```python
from build123d import *

# Parameters (mm, degrees)
BOX100_W                  = 187
BOX100_H                  = 3.4
BOX100_DEPTH              = 115
CYLINDER175_R             = 3
CYLINDER175_DEPTH         = 200
CYLINDER175_ROLL_ANGLE    = 90
CYLINDER176_R             = 3
CYLINDER176_DEPTH         = 200
CYLINDER176_ROLL_ANGLE    = 90
CYLINDER178_R             = 1.5
CYLINDER178_DEPTH         = 200
CYLINDER178_ROLL_ANGLE    = 90
CYLINDER177_R             = 1.5
CYLINDER177_DEPTH         = 200
CYLINDER177_ROLL_ANGLE    = 90
PAD090_DEPTH              = 55
BOX094_W                  = 5
BOX094_H                  = 176
BOX094_DEPTH              = 140
PAD091_DEPTH              = 55
BOX095_W                  = 6
BOX095_H                  = 176
BOX095_DEPTH              = 140
BOX093_W                  = 33
BOX093_H                  = 132
BOX093_DEPTH              = 54
BOX093_PLACEMENT_ANGLE    = 3
FILLET087_R               = 10
FILLET087_PLACEMENT_ANGLE = -3
BOX091_W                  = 18
BOX091_H                  = 17
BOX091_DEPTH              = 140
FILLET086_R               = 10
BOX090_W                  = 18
BOX090_H                  = 17
BOX090_DEPTH              = 140
FILLET085_R               = 10
BOX092_W                  = 182
BOX092_H                  = 16
BOX092_DEPTH              = 35
BOX097_W                  = 6
BOX097_H                  = 176
BOX097_DEPTH              = 80
BOX096_W                  = 5
BOX096_H                  = 176
BOX096_DEPTH              = 80
BOX088_W                  = 218
BOX088_H                  = 197
BOX088_DEPTH              = 10
FILLET083_R               = 10
FILLET084_R               = 10
CYLINDER172_R             = 2
CYLINDER172_DEPTH         = 300
CYLINDER172_PITCH_ANGLE   = 90
BOX099_W                  = 60
BOX099_H                  = 10
BOX099_DEPTH              = 10
FILLET089_R               = 4
FILLET090_R               = 10
FILLET091_R               = 10


with BuildPart() as cubo095:
    # Box100 → Box100 (new body)
    with BuildSketch(Plane(origin=(0, -44, 0), x_dir=(1, 0, 0), z_dir=(0, 0, 1))):
        with Locations((93.5, 1.7)):
            Rectangle(BOX100_W, BOX100_H)
    extrude(amount=BOX100_DEPTH)


with BuildPart() as obj1:
    # Cylinder175 → Cylinder175 (new body)
    with BuildSketch(Plane.XY):
        Circle(CYLINDER175_R)
    extrude(amount=CYLINDER175_DEPTH)


with BuildPart() as obj1_1:
    # Cylinder175 roll: moved
    add(obj1.part.rotate(Axis((0, 0, 0), (1, 0, 0)), CYLINDER175_ROLL_ANGLE))


with BuildPart() as obj1_2:
    # Cylinder175 placement: moved
    add(obj1_1.part.moved(Location((20, 165, 110))))


with BuildPart() as obj2:
    # Cylinder176 → Cylinder176 (new body)
    with BuildSketch(Plane.XY):
        Circle(CYLINDER176_R)
    extrude(amount=CYLINDER176_DEPTH)


with BuildPart() as obj2_1:
    # Cylinder176 roll: moved
    add(obj2.part.rotate(Axis((0, 0, 0), (1, 0, 0)), CYLINDER176_ROLL_ANGLE))


with BuildPart() as obj2_2:
    # Cylinder176 placement: moved
    add(obj2_1.part.moved(Location((160, 165, 110))))


with BuildPart() as obj3:
    # Cylinder178 → Cylinder178 (new body)
    with BuildSketch(Plane.XY):
        Circle(CYLINDER178_R)
    extrude(amount=CYLINDER178_DEPTH)


with BuildPart() as obj3_1:
    # Cylinder178 roll: moved
    add(obj3.part.rotate(Axis((0, 0, 0), (1, 0, 0)), CYLINDER178_ROLL_ANGLE))


with BuildPart() as obj3_2:
    # Cylinder178 placement: moved
    add(obj3_1.part.moved(Location((160, 154, 110))))


with BuildPart() as obj4:
    # Cylinder177 → Cylinder177 (new body)
    with BuildSketch(Plane.XY):
        Circle(CYLINDER177_R)
    extrude(amount=CYLINDER177_DEPTH)


with BuildPart() as obj4_1:
    # Cylinder177 roll: moved
    add(obj4.part.rotate(Axis((0, 0, 0), (1, 0, 0)), CYLINDER177_ROLL_ANGLE))


with BuildPart() as obj4_2:
    # Cylinder177 placement: moved
    add(obj4_1.part.moved(Location((20, 154, 110))))


with BuildPart() as pad090:
    # Sketch098 → Pad090 (new body)
    with BuildSketch(Plane(origin=(0, 0, 0), x_dir=(0, -1, 0), z_dir=(-1, 0, 0))):
        Polygon((-174.561249, 149.464645), (-73.728157, 149.464645), (-50.393822, 111), (-27.455967, 92.725647), (51.678024, 92.725647), (59.260941, 172), (-154.48703, 174.345367), align=None)
    extrude(amount=PAD090_DEPTH)


with BuildPart() as cut209:
    # Box094 → Box094 (new body)
    with BuildSketch(Plane(origin=(-15, -35, 0), x_dir=(1, 0, 0), z_dir=(0, 0, 1))):
        with Locations((2.5, 88)):
            Rectangle(BOX094_W, BOX094_H)
    extrude(amount=BOX094_DEPTH)

    # Cut209: cut Pad090
    add(pad090.part, mode=Mode.SUBTRACT)


with BuildPart() as pad091:
    # Sketch099 → Pad091 (new body)
    with BuildSketch(Plane(origin=(0, 0, 0), x_dir=(0, -1, 0), z_dir=(-1, 0, 0))):
        Polygon((-174.561249, 149.464645), (-73.728157, 149.464645), (-50.393822, 111), (-27.455967, 92.725647), (51.678024, 92.725647), (59.260941, 172), (-154.48703, 174.345367), align=None)
    extrude(amount=PAD091_DEPTH)


with BuildPart() as cut210:
    # Box095 → Box095 (new body)
    with BuildSketch(Plane(origin=(-15, -35, 0), x_dir=(1, 0, 0), z_dir=(0, 0, 1))):
        with Locations((3, 88)):
            Rectangle(BOX095_W, BOX095_H)
    extrude(amount=BOX095_DEPTH)

    # Cut210: cut Pad091
    add(pad091.part, mode=Mode.SUBTRACT)


with BuildPart() as cut210_1:
    # Cut210 placement: moved
    add(cut210.part.moved(Location((212, 0, 0))))


with BuildPart() as fillet104:
    # Box093 → Box093 (new body)
    with BuildSketch(Plane.XY):
        with Locations((16.5, 66)):
            Rectangle(BOX093_W, BOX093_H)
    extrude(amount=BOX093_DEPTH)


with BuildPart() as fillet104_1:
    # Box093 placement: moved
    add(fillet104.part.moved(Location((188, -32, 69))).rotate(Axis((188, -32, 69), (0, 0, 1)), BOX093_PLACEMENT_ANGLE))

    # Fillet087
    fillet087_edges = [fillet104_1.edges().sort_by_distance(p)[0] for p in [
        (204.477387, -31.136457, 69),
        (204.477387, -31.136457, 123),
        (197.569041, 100.682642, 69),
        (197.569041, 100.682642, 123),
    ]]
    fillet(fillet087_edges, radius=FILLET087_R)


with BuildPart() as fillet104_2:
    # Fillet087 placement: moved
    add(fillet104_1.part.moved(Location((0, 12, 0))).rotate(Axis((0, 12, 0), (0, 0, 1)), FILLET087_PLACEMENT_ANGLE))


with BuildPart() as fillet103:
    # Box091 → Box091 (new body)
    with BuildSketch(Plane(origin=(185, -48, 0), x_dir=(1, 0, 0), z_dir=(0, 0, 1))):
        with Locations((9, 8.5)):
            Rectangle(BOX091_W, BOX091_H)
    extrude(amount=BOX091_DEPTH)

    # Fillet086
    fillet086_edges = [fillet103.edges().sort_by_distance(p)[0] for p in [
        (203, -48, 70),
    ]]
    fillet(fillet086_edges, radius=FILLET086_R)


with BuildPart() as fillet102:
    # Box090 → Box090 (new body)
    with BuildSketch(Plane(origin=(-15, -48, 0), x_dir=(1, 0, 0), z_dir=(0, 0, 1))):
        with Locations((9, 8.5)):
            Rectangle(BOX090_W, BOX090_H)
    extrude(amount=BOX090_DEPTH)

    # Fillet085
    fillet085_edges = [fillet102.edges().sort_by_distance(p)[0] for p in [
        (-15, -48, 70),
    ]]
    fillet(fillet085_edges, radius=FILLET085_R)


with BuildPart() as cubo087:
    # Box092 → Box092 (new body)
    with BuildSketch(Plane(origin=(3, -48, 105), x_dir=(1, 0, 0), z_dir=(0, 0, 1))):
        with Locations((91, 8)):
            Rectangle(BOX092_W, BOX092_H)
    extrude(amount=BOX092_DEPTH)


with BuildPart() as cubo092:
    # Box097 → Box097 (new body)
    with BuildSketch(Plane(origin=(197, -35, 61), x_dir=(1, 0, 0), z_dir=(0, 0, 1))):
        with Locations((3, 88)):
            Rectangle(BOX097_W, BOX097_H)
    extrude(amount=BOX097_DEPTH)


with BuildPart() as cubo091:
    # Box096 → Box096 (new body)
    with BuildSketch(Plane(origin=(-15, -35, 61), x_dir=(1, 0, 0), z_dir=(0, 0, 1))):
        with Locations((2.5, 88)):
            Rectangle(BOX096_W, BOX096_H)
    extrude(amount=BOX096_DEPTH)


with BuildPart() as cut213:
    # Box088 → Box088 (new body)
    with BuildSketch(Plane(origin=(-15, -48, 140), x_dir=(1, 0, 0), z_dir=(0, 0, 1))):
        with Locations((109, 98.5)):
            Rectangle(BOX088_W, BOX088_H)
    extrude(amount=BOX088_DEPTH)

    # Fillet083
    fillet083_edges = [cut213.edges().sort_by_distance(p)[0] for p in [
        (-15, 149, 145),
        (203, 149, 145),
    ]]
    fillet(fillet083_edges, radius=FILLET083_R)

    # Fillet084
    fillet084_edges = [cut213.edges().sort_by_distance(p)[0] for p in [
        (-15, -48, 145),
        (203, -48, 145),
    ]]
    fillet(fillet084_edges, radius=FILLET084_R)

    # Fusion092: union Cubo092, Cubo091
    add(cubo092.part)
    add(cubo091.part)

    # Fusion093: union Fillet103, Fillet102, Cubo087
    add(fillet103.part)
    add(fillet102.part)
    add(cubo087.part)

    # Cut211: cut Fillet104
    add(fillet104_2.part, mode=Mode.SUBTRACT)

    # Cut212: cut Cut210
    add(cut210_1.part, mode=Mode.SUBTRACT)

    # Cut213: cut Cut209
    add(cut209.part, mode=Mode.SUBTRACT)


with BuildPart() as obj5:
    # Cylinder172 → Cylinder172 (new body)
    with BuildSketch(Plane.XY):
        Circle(CYLINDER172_R)
    extrude(amount=CYLINDER172_DEPTH)


with BuildPart() as obj5_1:
    # Cylinder172 pitch: moved
    add(obj5.part.rotate(Axis((0, 0, 0), (0, 1, 0)), CYLINDER172_PITCH_ANGLE))


with BuildPart() as obj5_2:
    # Cylinder172 placement: moved
    add(obj5_1.part.moved(Location((-54, 144, 135))))


with BuildPart() as top:
    # Box099 → Box099 (new body)
    with BuildSketch(Plane(origin=(64, 139, 130), x_dir=(1, 0, 0), z_dir=(0, 0, 1))):
        with Locations((30, 5)):
            Rectangle(BOX099_W, BOX099_H)
    extrude(amount=BOX099_DEPTH)

    # Fillet089
    fillet089_edges = [top.edges().sort_by_distance(p)[0] for p in [
        (94, 139, 130),
        (94, 149, 130),
    ]]
    fillet(fillet089_edges, radius=FILLET089_R)

    # Cut216: cut obj5
    add(obj5_2.part, mode=Mode.SUBTRACT)

    # Fusion094: union Cut213
    add(cut213.part)

    # Fillet090
    fillet090_edges = [top.edges().sort_by_distance(p)[0] for p in [
        (3, -40, 105),
    ]]
    fillet(fillet090_edges, radius=FILLET090_R)

    # Fillet091
    fillet091_edges = [top.edges().sort_by_distance(p)[0] for p in [
        (185, -40, 105),
    ]]
    fillet(fillet091_edges, radius=FILLET091_R)

    # Cut219: cut obj4
    add(obj4_2.part, mode=Mode.SUBTRACT)

    # Cut220: cut obj3
    add(obj3_2.part, mode=Mode.SUBTRACT)

    # Cut221: cut obj2
    add(obj2_2.part, mode=Mode.SUBTRACT)

    # Cut222: cut obj1
    add(obj1_2.part, mode=Mode.SUBTRACT)

    # Cut223: cut Cubo095
    add(cubo095.part, mode=Mode.SUBTRACT)


solid = top.part
```
Here's how the part is built. I have some questions about the finished solid (model axes, mm). A direction names the side the tool comes from. Coordinates: 2 decimals unless noted, no trailing zeros. Loops run counter-clockwise (first coordinate to the right, second up) from the corner with the lowest first, then second, coordinate; pieces in that order, holes last. Notation, with made-up numbers: (62, 3.5) -> (80, 3.5) arc R18 cw to (80, 15.5) -> close; hole circle Ø4 at (22, 24). An arc over 180 degrees is marked (long way). Return JSON: item names as keys, results as strings.
1) If we section it at D-D, the plane y = 61.5: Write out the boundary of the cut face in (x, z).
Results below:
{"outline": "(-15, 129.31) -> (-10, 129.31) -> (-10, 140) -> (197, 140) -> (197, 129.31) -> (203, 129.31) -> (203, 150) -> (-15, 150) -> close"}
2) Thinking about a two-plate mould opening in X: for faces 6 (the face through (200.15, 145.99, 145.07)), 7 (the face through (-12, -3, 92.726)), 8 (the face through (-12.15, -44.99, 76.05)), 9 (the face through (185, -36, 53)), which applies, +X half, -X half, draft (parallel to the pull), parting line (faces both ways), or undercut?
Results below:
{"face 6": "+X half", "face 7": "draft", "face 8": "-X half", "face 9": "undercut"}
3) For faces 1 (the face through (200, -35, 46)), 2 (the face through (6.01, -45.97, 102.15)), 3 (the face through (-10, 7, 116)), 4 (the face through (94, 139, 137)), 5 (the face through (161.3, -35, 108.7)), which set-ups out of +Z, -Z, +X, -X, +Y, -Y let a thin tool reach every point of the face, with its end or its side?
Results below:
{"face 1": "-Z, +X, +Y", "face 2": "-Z, +Y, -Y", "face 3": "-Z, +Y", "face 4": "-Z, +X, -X", "face 5": "+Y"}
4) If we section it at C-C, the plane y = 1.5: Write out the boundary of the cut face in (x, z).
Results below:
{"outline": "(-15, 92.73) -> (-10, 92.73) -> (-10, 140) -> (197, 140) -> (197, 123) -> (203, 123) -> (203, 150) -> (-15, 150) -> close"}
5) If we section it at B-B, the plane z = 36.5: Write out the boundary of the cut face in (x, y).
Results below:
{"outline": "(-15, -38) arc R10 ccw to (-5, -48) -> (3, -48) -> (3, -44) -> (0, -44) -> (0, -40.6) -> (3, -40.6) -> (3, -31) -> (-10, -31) -> (-10, -35) -> (-15, -35) -> close; (185, -48) -> (193, -48) arc R10 ccw to (203, -38) -> (203, -35) -> (197, -35) -> (197, -31) -> (185, -31) -> (185, -40.6) -> (187, -40.6) -> (187, -44) -> (185, -44) -> close"}
6) Will these pins go through, and if not, where does the flat tip stop? pin 1 (3 mm diameter, centred on x = 73, y = -45, fed in from -Z); pin 2 (3.5 mm diameter, centred on x = 20, z = 110, fed in from +Y); pin 3 (10 mm diameter, centred on x = 115.5, z = 98, fed in from -Y); pin 4 (1.2 mm diameter, centred on y = -46, z = 33, fed in from -X).
Results below:
{"pin 1": "z = 105", "pin 2": "y = -35", "pin 3": "through", "pin 4": "x = -11.73"}
7) If we section it at A-A, the plane x = 75: Write out the boundary of the cut face in (y, z), then the cut area to 3 significant figures.
Results below:
{"outline": "(-48, 105) -> (-44, 105) -> (-44, 115) -> (-40.6, 115) -> (-40.6, 105) -> (-32, 105) -> (-32, 140) -> (139, 140) -> (139, 134) arc R4 ccw to (143, 130) -> (145, 130) arc R4 ccw to (149, 134) -> (149, 150) -> (-48, 150) -> close; hole circle Ø4 at (144, 135)", "area": "2,580 mm²"}
8) I need wall thicknesses on line 1 (Z direction, x = 160, y = -45); line 2 (X direction, y = 14, z = 131); line 3 (Y direction, x = 18, z = 123.5). Which ranges of each line are inside material? Lowest first, please. Write a range as from..to.
Results below:
{"line 1": "105..108.5, 111.5..150", "line 2": "-15..-10, 197..203", "line 3": "-48..-32"}
